from build123d import *

# Parameters (mm, degrees)
SKETCH1_W           = 160
SKETCH1_H           = 85
SKETCH1_R           = 5
BOSS_EXTRUDE1_DEPTH = 5
SKETCH3_W           = 30
SKETCH3_H           = 85
CUT_EXTRUDE2_DEPTH  = 15
SKETCH5_R           = 2.55
CUT_EXTRUDE3_DEPTH  = 15
CHAMFER1_SIZE       = 10
SKETCH6_W           = 10
SKETCH6_H           = 5
BOSS_EXTRUDE2_DEPTH = 10
SKETCH7_R           = 2.55
CUT_EXTRUDE4_DEPTH  = 114.578166916
SKETCH8_R           = 2.55
CUT_EXTRUDE5_DEPTH  = 92.821838361


with BuildPart() as part:
    # Sketch1 → Boss-Extrude1 (new body)
    with BuildSketch(Plane.XY):
        Rectangle(SKETCH1_W, SKETCH1_H)
        Circle(SKETCH1_R, mode=Mode.SUBTRACT)
    extrude(amount=BOSS_EXTRUDE1_DEPTH)

    # Sketch3 → Cut-Extrude2 (cut)
    with BuildSketch(Plane.XY.offset(5)):
        with Locations((-65, 0)):
            Rectangle(SKETCH3_W, SKETCH3_H)
    extrude(amount=-CUT_EXTRUDE2_DEPTH, mode=Mode.SUBTRACT)

    # Sketch5 → Cut-Extrude3 (cut)
    with BuildSketch(Plane.XY.offset(5)):
        with Locations((65, 27.5)):
            Circle(SKETCH5_R)
        with Locations((50, 27.5)):
            Circle(SKETCH5_R)
        with Locations((35, 27.5)):
            Circle(SKETCH5_R)
        with Locations((20, 27.5)):
            Circle(SKETCH5_R)
        with Locations((5, 22.5)):
            Circle(SKETCH5_R)
        with Locations((-10, 22.5)):
            Circle(SKETCH5_R)
        with Locations((-25, 22.5)):
            Circle(SKETCH5_R)
        with Locations((-40, 22.5)):
            Circle(SKETCH5_R)
        with Locations((-40, -17.5)):
            Circle(SKETCH5_R)
    extrude(amount=-CUT_EXTRUDE3_DEPTH, mode=Mode.SUBTRACT)

    # Chamfer1
    chamfer1_edges = [part.edges().sort_by_distance(p)[0] for p in [
        (-50, -42.5, 2.5),
    ]]
    chamfer(chamfer1_edges, length=CHAMFER1_SIZE)

    # Sketch6 → Boss-Extrude2 (add)
    with BuildSketch(Plane(origin=(0, 0, 0), x_dir=(-1, 0, 0), z_dir=(0, 0, -1))):
        with Locations((-70, -40)):
            Rectangle(SKETCH6_W, SKETCH6_H)
        with Locations((25, -40)):
            Rectangle(SKETCH6_W, SKETCH6_H)
    boss_extrude2 = extrude(amount=BOSS_EXTRUDE2_DEPTH)

    # Sketch7 → Cut-Extrude4 (cut, through all)
    with BuildSketch(Plane(origin=(0, -37.5, 0), x_dir=(1, 0, 0), z_dir=(0, 1, 0))):
        with Locations(Location((70, 5, 0), (0, 0, 270))):
            Circle(SKETCH7_R)
        with Locations(Location((-25, 5, 0), (0, 0, 270))):
            Circle(SKETCH7_R)
    cut_extrude4 = extrude(amount=-CUT_EXTRUDE4_DEPTH, mode=Mode.SUBTRACT)

    # Mirror1: Boss-Extrude2 across plane
    add(boss_extrude2.mirror(Plane.ZX))

    # Mirror2: Cut-Extrude4 across plane
    add(cut_extrude4.mirror(Plane.ZX), mode=Mode.SUBTRACT)

    # Sketch8 → Cut-Extrude5 (cut, through all)
    with BuildSketch(Plane.XY.offset(5)):
        with Locations((75, 12.5)):
            Circle(SKETCH8_R)
        with Locations((75, -12.5)):
            Circle(SKETCH8_R)
    extrude(amount=-CUT_EXTRUDE5_DEPTH, mode=Mode.SUBTRACT)


solid = part.part
Read the model definition and answer for the solid it produces. Units are mm, in the model's axes. A direction names the side the tool comes from. Give positions to 0.01 mm unless a question says otherwise; leave off trailing zeros. Write each loop counter-clockwise with the first axis right and the second up, starting at its lowest first coordinate (ties: lowest second). Pieces come first, ordered by that corner, then holes. Notation, with made-up numbers: (40.25, 56) - (61.25, 56) arc R17 ccw to (61.25, 81) - close; hole circle Ø11 at (48.25, 58). An arc over 180 degrees is marked (long way). Answer in a Markdown table with one row per item. Add a question column.
Item 1: Flat-ended cylindrical pins translate along their axes: P1, Ø2.5, axis at y = -40, z = -4.5, coming from the +X side; P2, Ø4, axis at y = -40, z = -4.5, coming from the -X side; P3, Ø8, axis at x = -25, y = 22.5, coming from the -Z side; P4, Ø4.5, axis at x = 65, y = 27.5, coming from the -Z side. Find the tip coordinate at first contact, or state that the pin passes through.
Item 2: Section A-A, the plane y = 3 is taken. Write down the section's boundary in (x, z).
Item 3: Find the intervals of material crossed by L1, parallel to Y at x = 0, z = 1.85; L2, parallel to Z at x = -43.5, y = 27; L3, parallel to X at y = -33, z = 1, in increasing order.
Item 4: Section D-D, the plane y = 27.5 is taken. Write down the section's boundary in (x, z).
Item 5: Section C-C, the plane x = -10 is taken. Write down the section's boundary in (y, z).
Item 6: A tool of negligible diameter and unlimited length cuts with its end or side. For faces 1 (the face through (70, -40, -10)), 2 (the face through (-20, 40, -5)), 3 (the face through (75, 40, -5)), from which of +Z, -Z, +X, -X, +Y, -Y can it reach the whole face along a straight path? Write none if from no direction.
Item 7: Determine the mould class of faces 4 (the face through (-10.33, 25.03, 2.54)), 5 (the face through (-27.548, 22.612, 2.535)), 6 (the face through (65, -40, -5)) for opening direction Y: pulls with the +Y half, pulls with the -Y half, needs draft (parallel to the pull), parting line crosses it, or undercut.
Item 8: Section B-B, the plane x = -25 is taken. Write down the section's boundary in (y, z).
Recorded:
| question | item | result |
|---|---|---|
| 1 | P1 | stops at x = 75 |
| 1 | P2 | stops at x = -30 |
| 1 | P3 | stops at z = 0 |
| 1 | P4 | passes through |
| 2 | outline | (-50, 0) - (-4, 0) - (-4, 5) - (-50, 5) - close; (4, 0) - (80, 0) - (80, 5) - (4, 5) - close |
| 3 | L1 | y = -42.5 to -5, 5 to 42.5 |
| 3 | L2 | z = 0 to 5 |
| 3 | L3 | x = -49.5 to 80 |
| 4 | outline | (-50, 0) - (17.45, 0) - (17.45, 5) - (-50, 5) - close; (22.55, 0) - (32.45, 0) - (32.45, 5) - (22.55, 5) - close; (37.55, 0) - (47.45, 0) - (47.45, 5) - (37.55, 5) - close; (52.55, 0) - (62.45, 0) - (62.45, 5) - (52.55, 5) - close; (67.55, 0) - (80, 0) - (80, 5) - (67.55, 5) - close |
| 5 | outline | (-42.5, 0) - (19.95, 0) - (19.95, 5) - (-42.5, 5) - close; (25.05, 0) - (42.5, 0) - (42.5, 5) - (25.05, 5) - close |
| 6 | face 1 | -Z, +X, -X, +Y, -Y |
| 6 | face 2 | -Z, +Y, -Y |
| 6 | face 3 | -Z, +X, +Y, -Y |
| 7 | face 4 | undercut |
| 7 | face 5 | undercut |
| 7 | face 6 | needs draft |
| 8 | outline | (-42.5, -10) - (-37.5, -10) - (-37.5, -7.55) - (-42.5, -7.55) - close; (-42.5, -2.45) - (-37.5, -2.45) - (-37.5, 0) - (19.95, 0) - (19.95, 5) - (-42.5, 5) - close; (25.05, 0) - (37.5, 0) - (37.5, -2.45) - (42.5, -2.45) - (42.5, 5) - (25.05, 5) - close; (37.5, -10) - (42.5, -10) - (42.5, -7.55) - (37.5, -7.55) - close |
